from build123d import *

# Parameters (mm, degrees)
F0_W     = 223.52
F0_H     = 139.7
F0_R     = 1.5875
F1_DEPTH = 5.08
F2_R     = 3.175
F3_DEPTH = 50.8
F4_R     = 0.79375
F5_DEPTH = 51.562


with BuildPart() as f1:
    # F0 (on Top) → F1 (new body)
    with BuildSketch(Plane.XY):
        with Locations((-125.343207, 69.85)):
            Rectangle(F0_W, F0_H)
        with Locations((-176.778207, 34.925)):
            Circle(F0_R, mode=Mode.SUBTRACT)
        with Locations((-81.528207, 34.925)):
            Circle(F0_R, mode=Mode.SUBTRACT)
        with Locations((-176.778207, 104.775)):
            Circle(F0_R, mode=Mode.SUBTRACT)
        with Locations((-81.528207, 104.775)):
            Circle(F0_R, mode=Mode.SUBTRACT)
    extrude(amount=F1_DEPTH)

    # F2 (on face) → F3 (join)
    with BuildSketch(Plane.XY.offset(5.08)):
        Polygon((-229.483207, 139.7), (-237.103207, 139.7), (-237.103207, 132.08), (-237.103207, 124.46), (-237.103207, 15.24), (-237.103207, 7.62), (-237.103207, 0), (-229.483207, 0), (-221.863207, 0), (-125.343207, 0), (-28.823207, 0), (-21.203207, 0), (-13.583207, 0), (-13.583207, 7.62), (-13.583207, 15.24), (-13.583207, 124.46), (-13.583207, 132.08), (-13.583207, 139.7), (-21.203207, 139.7), (-28.823207, 139.7), (-125.343207, 139.7), (-221.863207, 139.7), align=None)
        with Locations((-230.727843, 7.62)):
            Circle(F2_R, mode=Mode.SUBTRACT)
        with Locations((-19.958571, 7.62)):
            Circle(F2_R, mode=Mode.SUBTRACT)
        with Locations((-230.727843, 132.08)):
            Circle(F2_R, mode=Mode.SUBTRACT)
        with BuildLine():
            Line((-232.023207, 15.24), (-232.023207, 124.46))
            Line((-232.023207, 124.46), (-229.901726, 124.46))
            ThreePointArc((-229.901726, 124.46), (-225.411598, 126.319872), (-223.551726, 130.81))
            Line((-223.551726, 130.81), (-223.551726, 134.62))
            Line((-223.551726, 134.62), (-125.343207, 134.62))
            Line((-125.343207, 134.62), (-27.134688, 134.62))
            Line((-27.134688, 134.62), (-27.134688, 130.81))
            ThreePointArc((-27.134688, 130.81), (-25.274816, 126.319872), (-20.784688, 124.46))
            Line((-20.784688, 124.46), (-18.663207, 124.46))
            Line((-18.663207, 124.46), (-18.663207, 15.24))
            Line((-18.663207, 15.24), (-20.784688, 15.24))
            ThreePointArc((-20.784688, 15.24), (-25.274816, 13.380128), (-27.134688, 8.89))
            Line((-27.134688, 8.89), (-27.134688, 5.08))
            Line((-27.134688, 5.08), (-125.343207, 5.08))
            Line((-125.343207, 5.08), (-223.551726, 5.08))
            Line((-223.551726, 5.08), (-223.551726, 8.89))
            ThreePointArc((-223.551726, 8.89), (-225.411598, 13.380128), (-229.901726, 15.24))
            Line((-229.901726, 15.24), (-232.023207, 15.24))
        make_face(mode=Mode.SUBTRACT)
        with Locations((-19.958571, 132.08)):
            Circle(F2_R, mode=Mode.SUBTRACT)
    extrude(amount=F3_DEPTH)

    # F4 (on face) → F5 (cut)
    with BuildSketch(Plane(origin=(-18.663207, 0, 0), x_dir=(0, -1, 0), z_dir=(-1, 0, 0))):
        with Locations((-82.55, 44.834881)):
            Circle(F4_R)
        with Locations((-57.15, 44.834881)):
            Circle(F4_R)
        with Locations((-82.55, 19.434881)):
            Circle(F4_R)
        with Locations((-57.15, 19.434881)):
            Circle(F4_R)
    extrude(amount=-F5_DEPTH, mode=Mode.SUBTRACT)


solid = f1.part
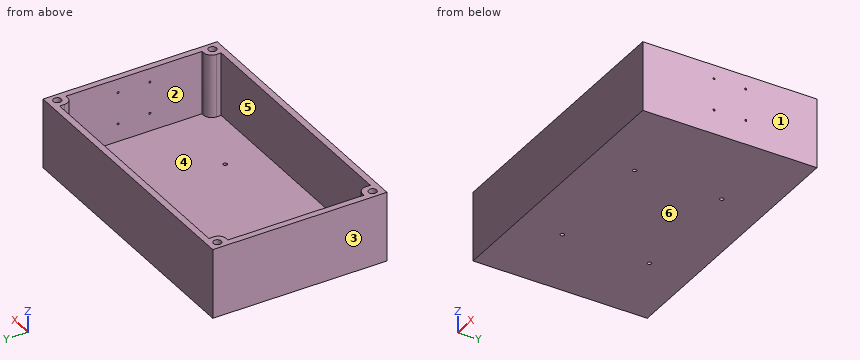
Geometry check sheet. Reference: the model listing, model coordinates, mm. Face numbers are marked on the shaded views. A direction names the side the tool comes from. Round coordinates to 2 decimals unless told otherwise and drop trailing zeros. Order: outer loops, then holes, each group sorted by start corner. A loop starts at its lowest first (then second) coordinate and runs counter-clockwise, first axis right, second up. Notation, with made-up numbers: M -11.5,-9 L 30.5,-9 A19 cw 30.5,2 Z; hole C 86,-19.75 d11. An arc over 180 degrees is marked long. Answer in a Markdown table with one row per item. Add a question column.
Item 1: Draft check along X on the marked faces 1, 2, 3 and 4. Enter one of: released by +X, released by -X, zero draft, split by the parting line, or undercut.
Item 2: Sectioned sample at B-B, the plane y = 121.5. Enter the section's corners in (x, z), plus the area to 3 significant figures.
Item 3: Depth check by flat-ended pin: pin 1 Ø3.5 at (x, y) = (-81.53, 104.78) entering from +Z; pin 2 Ø1.3 at (y, z) = (57.15, 44.83) entering from +X; pin 3 Ø3 at (x, y) = (-81.53, 34.92) entering from +Z. Enter the tip coordinate at first touch or a pass-through.
Item 4: Material ranges on L1, parallel to Y at x = -96, z = 23.5; L2, parallel to X at y = 24, z = 46; L3, parallel to X at y = 7, z = 13, recorded low to high. Write a range as [from, to].
Item 5: Set-up check for the marked faces 5 and 6: record each of +Z, -Z, +X, -X, +Y, -Y from which the full face is reachable in a straight line by a thin tool's end or side.
Item 6: Sectioned sample at C-C, the plane x = -197. Enter the section's corners in (y, z).
Item 7: Sectioned sample at A-A, the plane z = 37.5. Enter the section's corners in (x, y) (3 decimals).
Filled in:
| question | item | result |
|---|---|---|
| 1 | face 1 | released by +X |
| 1 | face 2 | undercut |
| 1 | face 3 | released by -X |
| 1 | face 4 | undercut |
| 2 | outline | M -237.1,0 L -13.58,0 L -13.58,55.88 L -18.66,55.88 L -18.66,5.08 L -232.02,5.08 L -232.02,55.88 L -237.1,55.88 Z |
| 2 | area | 1,650 mm² |
| 3 | pin 1 | stops at z = 5.08 |
| 3 | pin 2 | stops at x = -232.02 |
| 3 | pin 3 | passes through |
| 4 | L1 | y = [0, 5.08], [134.62, 139.7] |
| 4 | L2 | x = [-237.1, -232.02], [-18.66, -13.58] |
| 4 | L3 | x = [-237.1, -233.84], [-227.61, -223.55], [-27.13, -23.07], [-16.84, -13.58] |
| 5 | face 5 | +Z |
| 5 | face 6 | -Z, +X, -X, +Y, -Y |
| 6 | outline | M 0,0 L 139.7,0 L 139.7,55.88 L 134.62,55.88 L 134.62,5.08 L 5.08,5.08 L 5.08,55.88 L 0,55.88 Z |
| 7 | outline | M -237.103,0 L -13.583,0 L -13.583,139.7 L -237.103,139.7 Z; hole C -230.728,7.62 d6.35; hole C -230.728,132.08 d6.35; hole M -232.023,15.24 L -229.902,15.24 A6.35 cw -223.552,8.89 L -223.552,5.08 L -27.135,5.08 L -27.135,8.89 A6.35 cw -20.785,15.24 L -18.663,15.24 L -18.663,124.46 L -20.785,124.46 A6.35 cw -27.135,130.81 L -27.135,134.62 L -223.552,134.62 L -223.552,130.81 A6.35 cw -229.902,124.46 L -232.023,124.46 Z; hole C -19.959,7.62 d6.35; hole C -19.959,132.08 d6.35 |
